Study the drawing (mm; zero at the part's minimum x, y, z) and answer. Coordinates: 2 decimals unless noted, no trailing zeros. Order: outer loops, then holes, each group sorted by start corner. A loop starts at its lowest first (then second) coordinate and runs counter-clockwise, first axis right, second up.
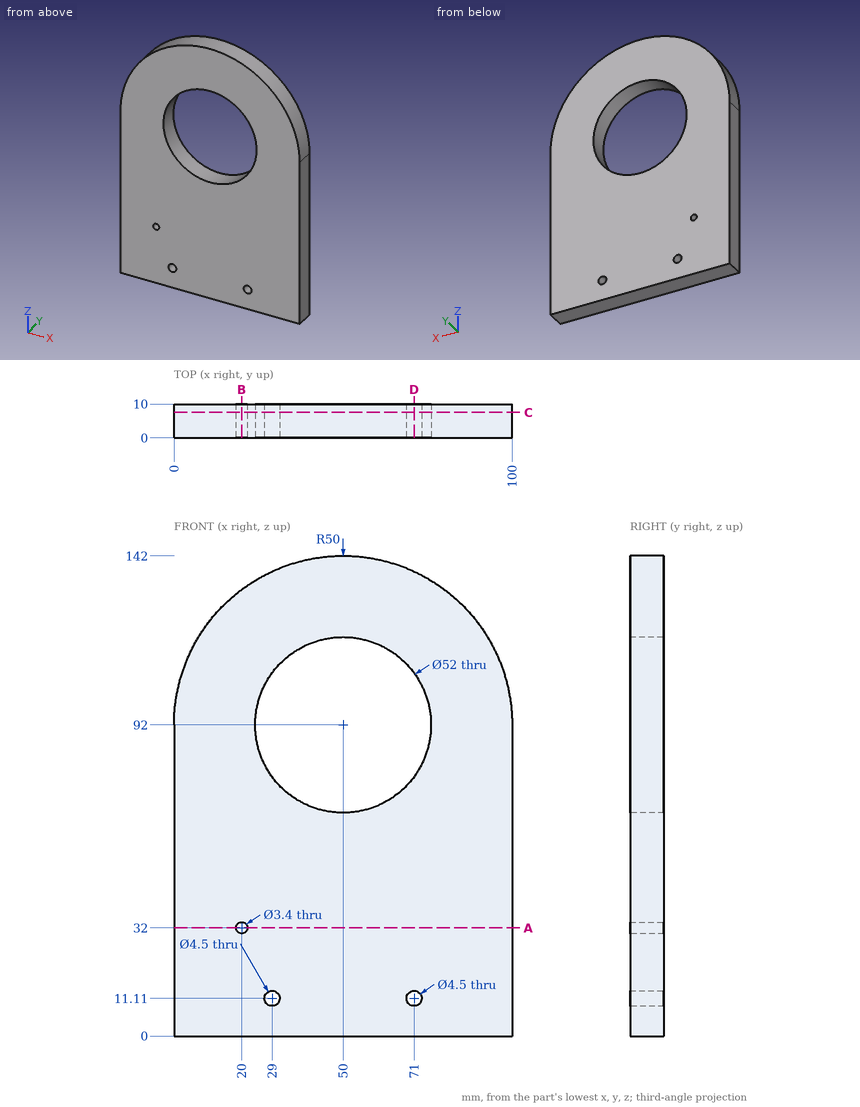
1) A cutting plane is placed at A-A, the plane z = 32. Determine the outline of the cut face in (x, y).
A:
outline: (0, 0) - (18.3, 0) - (18.3, 10) - (0, 10) - close; (21.7, 0) - (100, 0) - (100, 10) - (21.7, 10) - close
2) Flat-ended cylindrical pins translate along their axes: pin 1 Ø2 at (x, y) = (44.5, 2.5) entering from +Z; pin 2 Ø3 at (x, y) = (53.5, 6) entering from +Z. Find the tip coordinate at first contact, or state that the pin passes through.
A:
pin 1: stops at z = 141.8
pin 2: stops at z = 141.96
3) A cutting plane is placed at D-D, the plane x = 71. Determine the outline of the cut face in (y, z).
A:
outline: (0, 0) - (10, 0) - (10, 8.86) - (0, 8.86) - close; (0, 13.36) - (10, 13.36) - (10, 76.67) - (0, 76.67) - close; (0, 107.33) - (10, 107.33) - (10, 137.38) - (0, 137.38) - close
4) A cutting plane is placed at B-B, the plane x = 20. Determine the outline of the cut face in (y, z), and give its area (3 significant figures).
A:
outline: (0, 0) - (10, 0) - (10, 30.3) - (0, 30.3) - close; (0, 33.7) - (10, 33.7) - (10, 132) - (0, 132) - close
area: 1,290 mm2
5) Straight lines are drawn through the part: line 1 (X direction, y = 2.5, z = 11.11); line 2 (X direction, y = 6, z = 32); line 3 (X direction, y = 5.5, z = 91). For each, find the intervals that lie inside material, in ascending order.
A:
line 1: x = 0 to 26.75, 31.25 to 68.75, 73.25 to 100
line 2: x = 0 to 18.3, 21.7 to 100
line 3: x = 0 to 24.02, 75.98 to 100
6) A cutting plane is placed at C-C, the plane y = 7.5. Determine the outline of the cut face in (x, z).
A:
outline: (0, 0) - (100, 0) - (100, 92) arc R50 ccw to (0, 92) - close; hole circle Ø3.4 at (20, 32); hole circle Ø52 at (50, 92); hole circle Ø4.5 at (29, 11.11); hole circle Ø4.5 at (71, 11.11)
